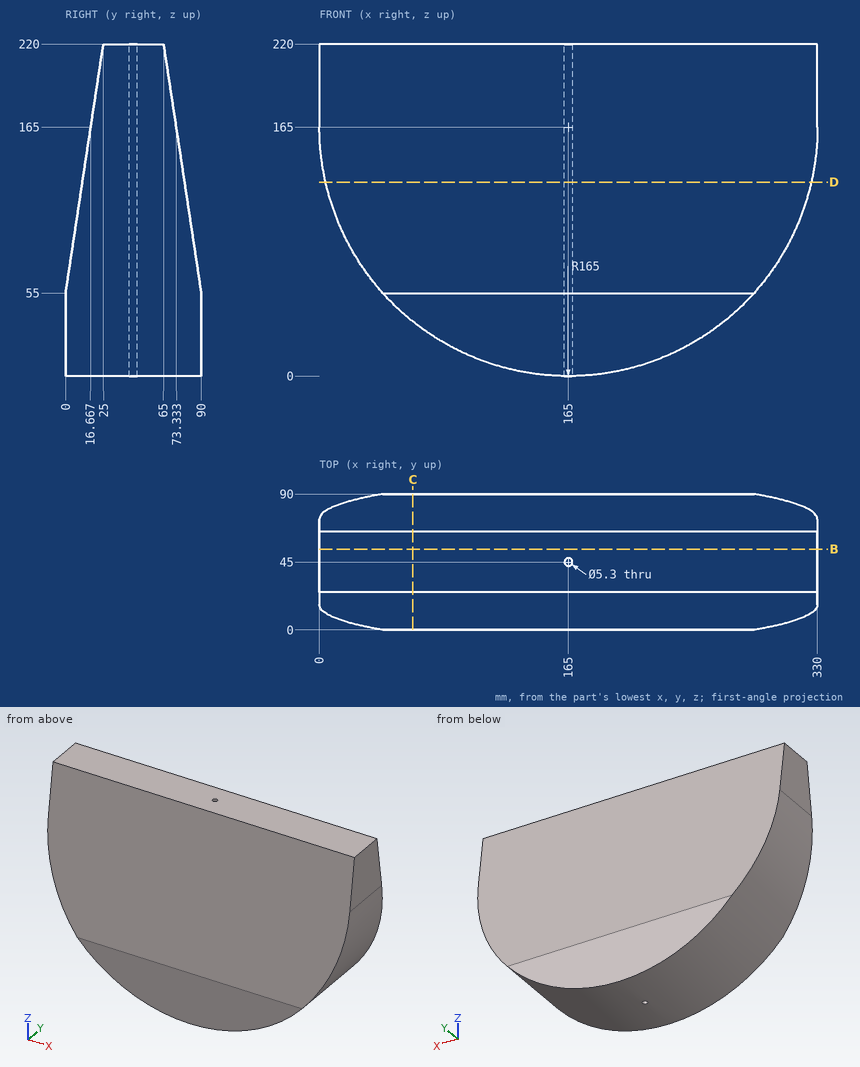
Study the drawing (mm; zero at the part's minimum x, y, z) and answer. Coordinates: 2 decimals unless noted, no trailing zeros. Order: outer loops, then holes, each group sorted by start corner. A loop starts at its lowest first (then second) coordinate and runs counter-clockwise, first axis right, second up. Notation, with made-up numbers: M 11,86 L 17,86 A15 cw 17,98 Z; hole C 23.5,71.5 d6. An arc over 180 degrees is marked long. Answer as a JSON object with one key per item and string values. Group by question number.
1. Section C-C on x = 62 is taken. Write down the section's boundary in (y, z), then the cut area to 3 significant figures.
2. Flat-ended cylindrical pins translate along their axes: P1, Ø8, axis at y = 79, z = 142, coming from the +X side; P2, Ø6, axis at x = 107, y = 70.5, coming from the -Z side; P3, Ø10, axis at x = 123, z = 157.5, coming from the +Y side. Find the tip coordinate at first contact, or state that the pin passes through.
3. Section D-D on z = 128.5 is taken. Write down the section's boundary in (x, y), then the cut area to 3 significant figures.
4. Straight lines are drawn through the part: line 1 (Y direction, x = 165, z = 119.5); line 2 (Y direction, x = 165, z = 80); line 3 (Y direction, x = 135, z = 71) (1 decimal). For each, find the intervals that lie inside material, in ascending order.
5. Section B-B on y = 53.5 is taken. Write down the section's boundary in (x, z), then the cut area to 3 significant figures.
Values follow:
{
 "1": {"outline": "M 0,36.1 L 90,36.1 L 90,55 L 65,220 L 25,220 L 0,55 Z", "area": "12,400 mm2"},
 "2": {"P1": "x = 328.78", "P2": "z = 9.44", "P3": "y = 75.23"},
 "3": {"outline": "M 4.09,11.14 L 325.91,11.14 L 325.91,78.86 L 4.09,78.86 Z; hole C 165,45 d5.3", "area": "21,800 mm2"},
 "4": {"line 1": "9.77 to 42.35, 47.65 to 80.23", "line 2": "3.79 to 42.35, 47.65 to 86.21", "line 3": "2.4 to 87.6"},
 "5": {"outline": "M 0,165 A165 ccw 330,165 L 330,220 L 0,220 Z", "area": "60,900 mm2"}
}
